from build123d import *

# Parameters (mm, degrees)
SKETCH1_R           = 3.2639
BOSS_EXTRUDE1_DEPTH = 3.175
SKETCH2_W           = 3.175
SKETCH2_H           = 12.7
BOSS_EXTRUDE2_DEPTH = 4.7625
SKETCH3_R           = 3.2639
CUT_EXTRUDE1_DEPTH  = 3.175
FILLET2_R           = 1.27


with BuildPart() as part:
    # Sketch1 → Boss-Extrude1 (new body)
    with BuildSketch(Plane.XY):
        with BuildLine():
            ThreePointArc((0, 6.35), (6.35, 0), (0, -6.35))
            Line((0, -6.35), (-9.017, -6.35))
            Line((-9.017, -6.35), (-9.017, 6.35))
            Line((-9.017, 6.35), (0, 6.35))
        make_face()
        Circle(SKETCH1_R, mode=Mode.SUBTRACT)
    extrude(amount=BOSS_EXTRUDE1_DEPTH)

    # Sketch2 → Boss-Extrude2 (add)
    with BuildSketch(Plane.XY.offset(3.175)):
        with Locations((-7.4295, 0)):
            Rectangle(SKETCH2_W, SKETCH2_H)
    extrude(amount=BOSS_EXTRUDE2_DEPTH)

    # Sketch3 → Cut-Extrude1 (cut)
    with BuildSketch(Plane.ZY.offset(9.017)):
        with Locations((2.38125, 0)):
            Circle(SKETCH3_R)
    extrude(amount=-CUT_EXTRUDE1_DEPTH, mode=Mode.SUBTRACT)

    # Fillet2
    fillet2_edges = [part.edges().sort_by_distance(p)[0] for p in [
        (-5.842, -4.757956423, 3.175),
        (-5.842, 4.757956423, 3.175),
    ]]
    fillet(fillet2_edges, radius=FILLET2_R)


solid = part.part
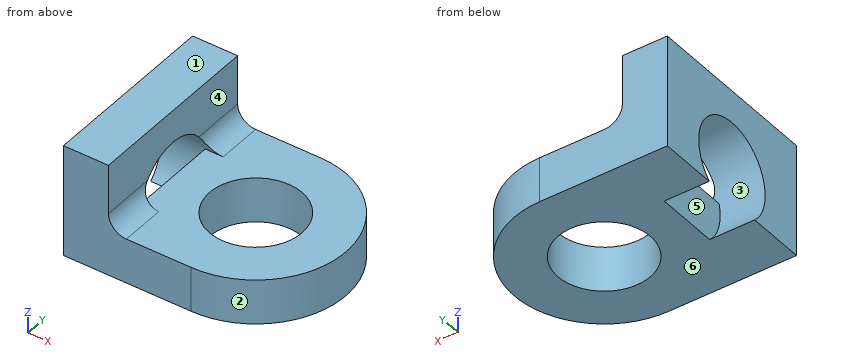
Model file for the job. Use its own axes, mm. Face numbers are marked on the shaded views. A direction names the side the tool comes from. Give positions to 0.01 mm unless a question says otherwise; leave off trailing zeros. Loops run counter-clockwise (first coordinate to the right, second up) from the corner with the lowest first, then second, coordinate; pieces in that order, holes last.
1) Tool access for the marked faces 4, 5 and 6: list every direction of +Z, -Z, +X, -X, +Y, -Y with a clear straight run to the whole face (end or side of a thin tool).
2) Saw through at A-A (y = 0). Count the separate pieces of the cut face and the enclosed holes in it, plus the area to 3 significant figures.
3) Wall check: line 1 (Z direction, x = 0, y = 5.75) (3 decimals); line 2 (X direction, y = 2.75, z = 6.5); line 3 (Y direction, x = -0.75, z = 1.25). Give the ranges that are in metal, low to high.
4) Flat gauge pins, fed straight in: pin 1 Ø6 at (x, y) = (-0.5, 1) entering from +Z (3 decimals); pin 2 Ø2.5 at (y, z) = (-1.5, 2) entering from -X; pin 3 Ø1.7 at (y, z) = (-0.5, 7) entering from +X. Where does each tip first touch, or does it go through?
5) Saw through at D-D (x = -1.5). Write the cut outline in (y, z) (3 decimals), plus the area to 3 significant figures.
6) Saw through at B-B (x = 0.75). Write the cut outline in (y, z) (3 decimals), plus the area to 3 significant figures.
7) Saw through at C-C (z = 2.25). Write the cut outline in (x, y), plus the area to 3 significant figures.
8) Pull direction Y, two halves, no side cores. Call the marked faces 1, 2 and 3: +Y half, -Y half, draft (parallel to the pull), parting line (faces both ways), or undercut.
Answer block:
1. face 4: +Z, +X, +Y, -Y
1. face 5: -X
1. face 6: -Z, +X, -X, +Y, -Y
2. separate pieces: 3
2. enclosed holes: 0
2. area: 25.3 mm2
3. line 1: z = 0 to 3.175
3. line 2: x = -9.02 to -5.84
3. line 3: y = -6.35 to -3.18, 3.18 to 6.35
4. pin 1: stops at z = 3.175
4. pin 2: stops at x = -5.84
4. pin 3: stops at x = -5.84
5. outline: (-6.35, 0) - (-2.899, 0) - (-2.899, 3.175) - (-6.35, 3.175) - close; (2.899, 0) - (6.35, 0) - (6.35, 3.175) - (2.899, 3.175) - close
5. area: 21.9 mm2
6. outline: (-6.306, 0) - (-3.177, 0) - (-3.177, 3.175) - (-6.306, 3.175) - close; (3.177, 0) - (6.306, 0) - (6.306, 3.175) - (3.177, 3.175) - close
6. area: 19.9 mm2
7. outline: (-9.02, -6.35) - (0, -6.35) arc R6.35 ccw to (0, 6.35) - (-9.02, 6.35) - (-9.02, 3.26) - (-5.84, 3.26) - (-5.84, -3.26) - (-9.02, -3.26) - close; hole circle Ø6.53 at (0, 0)
7. area: 124 mm2
8. face 1: draft
8. face 2: parting line
8. face 3: undercut
